Work out the finished part from the listing and answer in its coordinate system (mm). A direction names the side the tool comes from. Round coordinates to 2 decimals unless told otherwise and drop trailing zeros. Write each loop counter-clockwise with the first axis right and the second up, starting at its lowest first coordinate (ties: lowest second). Pieces come first, ordered by that corner, then holes.
1. A tool of negligible diameter and unlimited length cuts with its end or side. For faces 5 (the face through (-20.23, -1.53, 48.56)), 6 (the face through (-21, 0, -1)), 7 (the face through (-20.23, -150.87, 48.56)), from which of +Z, -Z, +X, -X, +Y, -Y can it reach the whole face along a straight path? Write none if from no direction.
2. Find section B-B (y = -57.5). Write down the section's boundary in (x, z) (3 decimals).
3. Flat-ended cylindrical pins translate along their axes: pin 1 Ø1 at (x, y) = (5, -102.5) entering from -Z; pin 2 Ø12 at (y, z) = (-84.5, 82) entering from -X; pin 3 Ø5 at (x, y) = (-38.5, -127) entering from -Z. Find the tip coordinate at first contact, or state that the pin passes through.
4. Determine the mould class of faces 1 (the face through (-18, -83.192, 100)), 2 (the face through (-23.495, -73, 97)), 3 (the face through (-21, -152.4, -1)), 4 (the face through (-39.93, -1.53, -41.07)) for opening direction Y: pulls with the +Y half, pulls with the -Y half, needs draft (parallel to the pull), parting line crosses it, or undercut.
5. Find section A-A (y = -20.5). Write down the section's boundary in (x, z), and give its area (3 significant figures).
6. Straight lines are drawn through the part: probe 1 along Z at (x, y) = (-20.5, -58); probe 2 along Z at (x, y) = (-18.5, -47.5); probe 3 along Y at (x, z) = (-30, -44). For each, find the intervals that lie inside material, in ascending order.
7. Find section C-C (z = 63). Write down the section's boundary in (x, y), and give its area (3 significant figures).
```python
from build123d import *

# Parameters (mm, degrees)
F1_DEPTH     = 152.4
F2_T1_DEPTH  = 159.9639298233
F2_T3_DEPTH  = 87.5512753886
F2_T5_DEPTH  = 105.6460143168
F2_T7_DEPTH  = 83.8431740092
F2_T9_DEPTH  = 66.9209927252
F2_T11_DEPTH = 67.7625979145
F2_T16_DEPTH = 5.08
F4_W         = 5.4661177176
F4_H         = 63.5
F7_DEPTH     = 3.175
F8_T1_DEPTH  = 142.24
F8_T3_DEPTH  = 87.5512753886
F8_T5_DEPTH  = 66.9209927252
F8_T7_DEPTH  = 52.3221869503
F8_T9_DEPTH  = 72.4030758235
F8_T11_DEPTH = 66.0406464801
F8_T16_DEPTH = 5.08
F8_T22_DEPTH = 5.08
F8_T28_DEPTH = 5.08
F8_T34_DEPTH = 5.08
F8_T38_ANGLE = 89.746481368


# Not quite as in the source:
# - a fillet or chamfer that OpenCascade refuses, or shapes differently, is made with other operations: its cross-section is extruded or revolved along the edge and cut away or added


with BuildPart() as f1:
    # F0 (on Front) → F1 (new body)
    with BuildSketch(Plane.XZ):
        Polygon((17.4287217617, 50.174562376), (-58.7712782383, 49.8373953771), (-58.7712782383, -30.0714519408), (-24.3801281386, -53.3360523395), (-17.9739344996, -53.3360523395), (17.4287217617, -30.0714519408), align=None)
    extrude(amount=F1_DEPTH)

    # F2: fillet of radius 5.08 on 6 edges, made by hand

    # F2_s2 → F2_t1 (cut)
    with BuildSketch(Plane.XZ.offset(-12.6439298233)):
        with BuildLine():
            ThreePointArc((-53.7137558182, 49.859773719), (-57.2913189399, 48.3639700613), (-58.7712782383, 44.7798234478))
            Line((-58.7712782383, 44.7798234478), (-58.7712782383, 49.8373953771))
            Line((-58.7712782383, 49.8373953771), (-53.7137558182, 49.859773719))
        make_face()
    extrude(amount=F2_T1_DEPTH, mode=Mode.SUBTRACT)

    # F2_s4 → F2_t3 (cut)
    with BuildSketch(Plane.XY.offset(-42.7714519408)):
        with BuildLine():
            ThreePointArc((-58.7712782383, -147.32), (-57.2833806867, -150.9121024484), (-53.6912782383, -152.4))
            Line((-53.6912782383, -152.4), (-58.7712782383, -152.4))
            Line((-58.7712782383, -152.4), (-58.7712782383, -147.32))
        make_face()
    extrude(amount=F2_T3_DEPTH, mode=Mode.SUBTRACT)

    # F2_s6 → F2_t5 (cut)
    with BuildSketch(Plane.XY.offset(-42.7714519408)):
        with BuildLine():
            ThreePointArc((17.4287217617, -147.32), (15.9408242101, -150.9121024484), (12.3487217617, -152.4))
            Line((12.3487217617, -152.4), (17.4287217617, -152.4))
            Line((17.4287217617, -152.4), (17.4287217617, -147.32))
        make_face()
    extrude(amount=F2_T5_DEPTH, mode=Mode.SUBTRACT)

    # F2_s8 → F2_t7 (cut)
    with BuildSketch(Plane(origin=(30.3502624567, 0, 0.1342927416), x_dir=(0, 1, 0), z_dir=(-0.9999902109, 0, -0.0044247205))):
        with BuildLine():
            ThreePointArc((-147.32, -50.0969539894), (-150.9121024484, -48.6090564378), (-152.4, -45.0169539894))
            Line((-152.4, -45.0169539894), (-152.4, -50.0969539894))
            Line((-152.4, -50.0969539894), (-147.32, -50.0969539894))
        make_face()
    extrude(amount=F2_T7_DEPTH, mode=Mode.SUBTRACT)

    # F2_s10 → F2_t9 (cut)
    with BuildSketch(Plane(origin=(-36.8834278428, 0, 24.9505529071), x_dir=(0, 1, 0), z_dir=(0.8282834259, 0, -0.5603093489))):
        with BuildLine():
            ThreePointArc((-147.32, -57.8377818767), (-150.9121024484, -56.3498843251), (-152.4, -52.7577818767))
            Line((-152.4, -52.7577818767), (-152.4, -57.8377818767))
            Line((-152.4, -57.8377818767), (-147.32, -57.8377818767))
        make_face()
    extrude(amount=F2_T9_DEPTH, mode=Mode.SUBTRACT)

    # F2_s12 → F2_t11 (cut)
    with BuildSketch(Plane(origin=(-47.6451540495, 0, -31.3096695828), x_dir=(0, 1, 0), z_dir=(0.8357055045, 0, 0.549177849))):
        with BuildLine():
            ThreePointArc((-147.32, -34.7023458418), (-150.9121024484, -33.2144482902), (-152.4, -29.6223458418))
            Line((-152.4, -29.6223458418), (-152.4, -34.7023458418))
            Line((-152.4, -34.7023458418), (-147.32, -34.7023458418))
        make_face()
    extrude(amount=F2_T11_DEPTH, mode=Mode.SUBTRACT)


with BuildPart() as f2_tool14:
    # F2_s15 → F2_t16 (new body)
    with BuildSketch(Plane.XZ.offset(147.32)):
        Polygon((-53.6912782383, 44.7798234478), (-53.7137558182, 49.859773719), (-58.7712782383, 49.8373953771), (-58.7712782383, 44.7798234478), align=None)
    extrude(amount=F2_T16_DEPTH)

    # F2_s17 → F2_t18 (revolve, cut)
    with BuildSketch(Plane(origin=(-53.6912782383, -147.32, 44.7798234478), x_dir=(0.7086694294, 0, -0.7055406719), z_dir=(-0.7055406719, 0, -0.7086694294))):
        with BuildLine():
            ThreePointArc((0, -5.08), (5.08, 0), (0, 5.08))
            Line((0, 5.08), (0, -5.08))
        make_face()
    revolve(axis=Axis((-53.6912782383, -147.32, 44.7798234478), (0, -1, 0)), mode=Mode.SUBTRACT)


with BuildPart() as f1_1:
    add(f1.part)

    # F2_t13: cut F2_tool14
    add(f2_tool14.part, mode=Mode.SUBTRACT)

    # F4 (on offset) → F5 (revolve)
    with BuildSketch(Plane.YZ.offset(-20.32)):
        with Locations((-85.7021328023, 81.609773719)):
            Rectangle(F4_W, F4_H)
    revolve(axis=Axis((-20.32, -88.4351916611, 88.4142501174), (0, 0, 1)))

    # F6 (on offset) → F7 (join, symmetric)
    with BuildSketch(Plane.YZ.offset(-20.32)):
        Polygon((-46.0359752178, 96.2450280786), (-83.1919163465, 113.4468540549), (-83.1919163465, 86.9560390711), align=None)
    extrude(amount=F7_DEPTH, both=True)

    # F8: fillet of radius 5.08 on 8 edges, made by hand

    # F8_s2 → F8_t1 (cut)
    with BuildSketch(Plane.XZ.offset(5.08)):
        with BuildLine():
            ThreePointArc((12.3262441818, 50.1519851181), (15.9328683752, 48.6720755484), (17.4287217617, 45.0720348468))
            Line((17.4287217617, 45.0720348468), (17.4287217617, 50.174562376))
            Line((17.4287217617, 50.174562376), (12.3262441818, 50.1519851181))
        make_face()
        with BuildLine():
            ThreePointArc((15.1385452344, -31.5764249394), (16.8196670332, -29.7428967724), (17.4287217617, -27.3310409766))
            Line((17.4287217617, -27.3310409766), (17.4287217617, -30.0714519408))
            Line((17.4287217617, -30.0714519408), (15.1385452344, -31.5764249394))
        make_face()
    extrude(amount=F8_T1_DEPTH, mode=Mode.SUBTRACT)

    # F8_s4 → F8_t3 (cut)
    with BuildSketch(Plane.XY.offset(-42.7714519408)):
        with BuildLine():
            ThreePointArc((-58.7712782383, -5.08), (-57.2833806867, -1.4878975516), (-53.6912782383, 0))
            Line((-53.6912782383, 0), (-58.7712782383, 0))
            Line((-58.7712782383, 0), (-58.7712782383, -5.08))
        make_face()
    extrude(amount=F8_T3_DEPTH, mode=Mode.SUBTRACT)

    # F8_s6 → F8_t5 (cut)
    with BuildSketch(Plane(origin=(-36.8834278428, 0, 24.9505529071), x_dir=(0, 1, 0), z_dir=(0.8282834259, 0, -0.5603093489))):
        with BuildLine():
            ThreePointArc((-5.08, -57.8377818767), (-1.4878975516, -56.3498843251), (0, -52.7577818767))
            Line((0, -52.7577818767), (0, -57.8377818767))
            Line((0, -57.8377818767), (-5.08, -57.8377818767))
        make_face()
    extrude(amount=F8_T5_DEPTH, mode=Mode.SUBTRACT)

    # F8_s8 → F8_t7 (cut)
    with BuildSketch(Plane(origin=(-47.6451540495, 0, -31.3096695828), x_dir=(0, 1, 0), z_dir=(0.8357055045, 0, 0.549177849))):
        with BuildLine():
            ThreePointArc((-5.08, -34.7023458418), (-1.4878975516, -33.2144482902), (0, -29.6223458418))
            Line((0, -29.6223458418), (0, -34.7023458418))
            Line((0, -34.7023458418), (-5.08, -34.7023458418))
        make_face()
    extrude(amount=F8_T7_DEPTH, mode=Mode.SUBTRACT)

    # F8_s10 → F8_t9 (cut)
    with BuildSketch(Plane.XY.offset(-27.3310409766)):
        with BuildLine():
            ThreePointArc((17.4287217617, -5.08), (15.9408242101, -1.4878975516), (12.3487217617, 0))
            Line((12.3487217617, 0), (17.4287217617, 0))
            Line((17.4287217617, 0), (17.4287217617, -5.08))
        make_face()
    extrude(amount=F8_T9_DEPTH, mode=Mode.SUBTRACT)

    # F8_s12 → F8_t11 (cut)
    with BuildSketch(Plane(origin=(12.5479091987, 0, 0.055521534), x_dir=(0, 1, 0), z_dir=(-0.9999902109, 0, -0.0044247205))):
        with BuildLine():
            ThreePointArc((-5.08, -50.0969539894), (-1.4878975516, -48.6090564378), (0, -45.0169539894))
            Line((0, -45.0169539894), (0, -50.0969539894))
            Line((0, -50.0969539894), (-5.08, -50.0969539894))
        make_face()
    extrude(amount=F8_T11_DEPTH, mode=Mode.SUBTRACT)


with BuildPart() as f8_tool14:
    # F8_s15 → F8_t16 (new body)
    with BuildSketch(Plane.XZ.offset(147.32)):
        Polygon((12.3487217617, -27.3310409766), (15.1385452344, -31.5764249394), (17.4287217617, -30.0714519408), (17.4287217617, -27.3310409766), align=None)
    extrude(amount=F8_T16_DEPTH)

    # F8_s17 → F8_t18 (revolve, cut)
    with BuildSketch(Plane(origin=(12.3487217617, -147.32, -27.3310409766), x_dir=(-0.8801073369, 0, 0.4747747629), z_dir=(0.4747747629, 0, 0.8801073369))):
        with BuildLine():
            ThreePointArc((0, -5.08), (5.08, 0), (0, 5.08))
            Line((0, 5.08), (0, -5.08))
        make_face()
    revolve(axis=Axis((12.3487217617, -147.32, -27.3310409766), (0, -1, 0)), mode=Mode.SUBTRACT)


with BuildPart() as f1_2:
    add(f1_1.part)

    # F8_t13: cut F8_tool14
    add(f8_tool14.part, mode=Mode.SUBTRACT)


with BuildPart() as f8_tool20:
    # F8_s21 → F8_t22 (new body)
    with BuildSketch(Plane.XZ.offset(147.32)):
        Polygon((12.3487217617, 45.0720348468), (12.3262441818, 50.1519851181), (17.4287217617, 50.174562376), (17.4287217617, 45.0720348468), align=None)
    extrude(amount=F8_T22_DEPTH)

    # F8_s23 → F8_t24 (revolve, cut)
    with BuildSketch(Plane(origin=(12.3487217617, -147.32, 45.0720348468), x_dir=(-0.7055406719, 0, -0.7086694294), z_dir=(-0.7086694294, 0, 0.7055406719))):
        with BuildLine():
            ThreePointArc((0, -5.08), (5.08, 0), (0, 5.08))
            Line((0, 5.08), (0, -5.08))
        make_face()
    revolve(axis=Axis((12.3487217617, -147.32, 45.0720348468), (0, -1, 0)), mode=Mode.SUBTRACT)


with BuildPart() as f1_3:
    add(f1_2.part)

    # F8_t19: cut F8_tool20
    add(f8_tool20.part, mode=Mode.SUBTRACT)


with BuildPart() as f8_tool26:
    # F8_s27 → F8_t28 (new body)
    with BuildSketch(Plane.XZ.offset(5.08)):
        Polygon((12.3487217617, 45.0720348468), (12.3262441818, 50.1519851181), (17.4287217617, 50.174562376), (17.4287217617, 45.0720348468), align=None)
    extrude(amount=-F8_T28_DEPTH)

    # F8_s29 → F8_t30 (revolve, cut)
    with BuildSketch(Plane(origin=(12.3487217617, -5.08, 45.0720348468), x_dir=(-0.7055406719, 0, -0.7086694294), z_dir=(0.7086694294, 0, -0.7055406719))):
        with BuildLine():
            ThreePointArc((0, -5.08), (5.08, 0), (0, 5.08))
            Line((0, 5.08), (0, -5.08))
        make_face()
    revolve(axis=Axis((12.3487217617, -5.08, 45.0720348468), (0, 1, 0)), mode=Mode.SUBTRACT)


with BuildPart() as f1_4:
    add(f1_3.part)

    # F8_t25: cut F8_tool26
    add(f8_tool26.part, mode=Mode.SUBTRACT)


with BuildPart() as f8_tool32:
    # F8_s33 → F8_t34 (new body)
    with BuildSketch(Plane.XZ.offset(5.08)):
        Polygon((12.3487217617, -27.3310409766), (15.1385452344, -31.5764249394), (17.4287217617, -30.0714519408), (17.4287217617, -27.3310409766), align=None)
    extrude(amount=-F8_T34_DEPTH)

    # F8_s35 → F8_t36 (revolve, cut)
    with BuildSketch(Plane(origin=(12.3487217617, -5.08, -27.3310409766), x_dir=(-0.8801073369, 0, 0.4747747629), z_dir=(-0.4747747629, 0, -0.8801073369))):
        with BuildLine():
            ThreePointArc((0, -5.08), (5.08, 0), (0, 5.08))
            Line((0, 5.08), (0, -5.08))
        make_face()
    revolve(axis=Axis((12.3487217617, -5.08, -27.3310409766), (0, 1, 0)), mode=Mode.SUBTRACT)


with BuildPart() as f1_5:
    add(f1_4.part)

    # F8_t31: cut F8_tool32
    add(f8_tool32.part, mode=Mode.SUBTRACT)

    # F8_s37 → F8_t38 (revolve, cut)
    with BuildSketch(Plane.XY.offset(44.7798234479)):
        with BuildLine():
            ThreePointArc((-58.7712782383, -5.08), (-57.2833806867, -1.4878975516), (-53.6912782383, 0))
            Line((-53.6912782383, 0), (-58.7712782383, 0))
            Line((-58.7712782383, 0), (-58.7712782383, -5.08))
        make_face()
    revolve(axis=Axis((-53.6912782384, 0, 44.7798234479), (0, 1, 0)), revolution_arc=F8_T38_ANGLE, mode=Mode.SUBTRACT)


solid = f1_5.part
```
Worked answers:
1. face 5: +Z, -X, +Y
1. face 6: +Z, -Z, +X, -X, +Y
1. face 7: +Z, -X, -Y
2. outline: (-58.771, -30.071) - (-24.38, -53.336) - (-17.974, -53.336) - (15.139, -31.576) arc R5.08 ccw to (17.429, -27.331) - (17.429, 45.072) arc R5.08 ccw to (12.326, 50.152) - (-53.714, 49.86) arc R5.08 ccw to (-58.771, 44.78) - close; (-23.495, 93.379) - (-17.145, 93.379) - (-17.145, 101.552) - (-23.495, 101.552) - close
3. pin 1: stops at z = -38.57
3. pin 2: stops at x = -25.79
3. pin 3: stops at z = -45.48
4. face 1: undercut
4. face 2: needs draft
4. face 3: pulls with the -Y half
4. face 4: pulls with the +Y half
5. outline: (-58.77, -30.07) - (-24.38, -53.34) - (-17.97, -53.34) - (15.14, -31.58) arc R5.08 ccw to (17.43, -27.33) - (17.43, 45.07) arc R5.08 ccw to (12.33, 50.15) - (-53.71, 49.86) arc R5.08 ccw to (-58.77, 44.78) - close
5. area: 7,050 mm2
6. probe 1: z = -53.34 to 50.01, 93.25 to 101.78
6. probe 2: z = -53.34 to 50.02, 95.88 to 96.92
6. probe 3: y = -152.38 to -0.02
7. outline: circle Ø10.93 at (-20.32, -88.44)
7. area: 93.9 mm2
